```python
from build123d import *

# Parameters (mm, degrees)
SKETCH1_W            = 48
SKETCH1_H            = 53
BOSS_EXTRUDE1_DEPTH  = 10
SKETCH2_W            = 48
SKETCH2_H            = 5.616325
BOSS_EXTRUDE2_DEPTH  = 33.1917878
SKETCH4_W            = 4
SKETCH4_H            = 10
BOSS_EXTRUDE4_DEPTH  = 40
SKETCH5_W            = 48
SKETCH5_H            = 10.8609375
BOSS_EXTRUDE5_DEPTH  = 23.1917878
SKETCH6_W            = 48
SKETCH6_H            = 5
BOSS_EXTRUDE6_DEPTH  = 42.3
SKETCH7_W            = 12.8082122
SKETCH7_H            = 16.4772625
BOSS_EXTRUDE7_DEPTH  = 48
CUT_EXTRUDE1_REACH   = 84.426
SKETCH8_R            = 11.5
SKETCH8_R_2          = 1.5
FILLET1_R            = 10
FILLET2_R            = 4
SKETCH9_W            = 5
SKETCH9_H            = 16.4772625
BOSS_EXTRUDE9_DEPTH  = 48
CUT_EXTRUDE2_DEPTH   = 6
SKETCH11_R           = 1.9304
CUT_EXTRUDE3_DEPTH   = 6
BOSS_EXTRUDE11_DEPTH = 3
SKETCH14_W           = 45
SKETCH14_H           = 17
CUT_EXTRUDE4_DEPTH   = 4
CUT_EXTRUDE5_REACH   = 88.925


with BuildPart() as part:
    # Sketch1 → Boss-Extrude1 (new body)
    with BuildSketch(Plane.XY):
        with Locations((24, 26.5)):
            Rectangle(SKETCH1_W, SKETCH1_H)
    extrude(amount=BOSS_EXTRUDE1_DEPTH)

    # Sketch2 → Boss-Extrude2 (add)
    with BuildSketch(Plane(origin=(0, 0, 0), x_dir=(-1, 0, 0), z_dir=(0, 0, -1))):
        with Locations((-24, -2.8081625)):
            Rectangle(SKETCH2_W, SKETCH2_H)
    extrude(amount=-BOSS_EXTRUDE2_DEPTH)

    # Sketch4 → Boss-Extrude4 (add)
    with BuildSketch(Plane.XY.offset(10)):
        with Locations((2, 48)):
            Rectangle(SKETCH4_W, SKETCH4_H)
        with Locations((46, 48)):
            Rectangle(SKETCH4_W, SKETCH4_H)
    extrude(amount=BOSS_EXTRUDE4_DEPTH)

    # Sketch5 → Boss-Extrude5 (add)
    with BuildSketch(Plane.XY.offset(10)):
        with Locations((24, 5.43046875)):
            Rectangle(SKETCH5_W, SKETCH5_H)
    extrude(amount=BOSS_EXTRUDE5_DEPTH)

    # Sketch6 → Boss-Extrude6 (add)
    with BuildSketch(Plane.XZ.offset(5.616325)):
        with Locations((24, 30.6917878)):
            Rectangle(SKETCH6_W, SKETCH6_H)
    extrude(amount=BOSS_EXTRUDE6_DEPTH)

    # Sketch7 → Boss-Extrude7 (add)
    with BuildSketch(Plane.ZY):
        with Locations((-6.4041061, 2.62230625)):
            Rectangle(SKETCH7_W, SKETCH7_H)
    extrude(amount=-BOSS_EXTRUDE7_DEPTH)

    # Sketch8 → Cut-Extrude1 (cut, up to next)
    with BuildSketch(Plane(origin=(0, 0, 28.1917878), x_dir=(-1, 0, 0), z_dir=(0, 0, -1)), mode=Mode.PRIVATE) as cut_extrude1_sk1:
        with Locations((-24, -26.616325)):
            Circle(SKETCH8_R)
    cut_extrude1_tool1 = extrude(cut_extrude1_sk1.sketch, amount=-CUT_EXTRUDE1_REACH, mode=Mode.PRIVATE) & part.part
    # Sketch8 → Cut-Extrude1 (cut, up to next)
    with BuildSketch(Plane(origin=(0, 0, 28.1917878), x_dir=(-1, 0, 0), z_dir=(0, 0, -1)), mode=Mode.PRIVATE) as cut_extrude1_sk2:
        with Locations((-39.5, -11.116325)):
            Circle(SKETCH8_R_2)
    cut_extrude1_tool2 = extrude(cut_extrude1_sk2.sketch, amount=-CUT_EXTRUDE1_REACH, mode=Mode.PRIVATE) & part.part
    # Sketch8 → Cut-Extrude1 (cut, up to next)
    with BuildSketch(Plane(origin=(0, 0, 28.1917878), x_dir=(-1, 0, 0), z_dir=(0, 0, -1)), mode=Mode.PRIVATE) as cut_extrude1_sk3:
        with Locations((-39.5, -42.116325)):
            Circle(SKETCH8_R_2)
    cut_extrude1_tool3 = extrude(cut_extrude1_sk3.sketch, amount=-CUT_EXTRUDE1_REACH, mode=Mode.PRIVATE) & part.part
    # Sketch8 → Cut-Extrude1 (cut, up to next)
    with BuildSketch(Plane(origin=(0, 0, 28.1917878), x_dir=(-1, 0, 0), z_dir=(0, 0, -1)), mode=Mode.PRIVATE) as cut_extrude1_sk4:
        with Locations((-8.5, -11.116325)):
            Circle(SKETCH8_R_2)
    cut_extrude1_tool4 = extrude(cut_extrude1_sk4.sketch, amount=-CUT_EXTRUDE1_REACH, mode=Mode.PRIVATE) & part.part
    # Sketch8 → Cut-Extrude1 (cut, up to next)
    with BuildSketch(Plane(origin=(0, 0, 28.1917878), x_dir=(-1, 0, 0), z_dir=(0, 0, -1)), mode=Mode.PRIVATE) as cut_extrude1_sk5:
        with Locations((-8.5, -42.116325)):
            Circle(SKETCH8_R_2)
    cut_extrude1_tool5 = extrude(cut_extrude1_sk5.sketch, amount=-CUT_EXTRUDE1_REACH, mode=Mode.PRIVATE) & part.part
    add(cut_extrude1_tool1.solids().sort_by_distance((24, -26.616325, 28.191788))[0], mode=Mode.SUBTRACT)
    add(cut_extrude1_tool2.solids().sort_by_distance((39.5, -11.116325, 28.191788))[0], mode=Mode.SUBTRACT)
    add(cut_extrude1_tool3.solids().sort_by_distance((39.5, -42.116325, 28.191788))[0], mode=Mode.SUBTRACT)
    add(cut_extrude1_tool4.solids().sort_by_distance((8.5, -11.116325, 28.191788))[0], mode=Mode.SUBTRACT)
    add(cut_extrude1_tool5.solids().sort_by_distance((8.5, -42.116325, 28.191788))[0], mode=Mode.SUBTRACT)

    # Fillet1
    fillet1_edges = [part.edges().sort_by_distance(p)[0] for p in [
        (24, 10.8609375, 0),
    ]]
    fillet(fillet1_edges, radius=FILLET1_R)

    # Fillet2
    fillet2_edges = [part.edges().sort_by_distance(p)[0] for p in [
        (2, 43, 10),
        (46, 43, 10),
    ]]
    fillet(fillet2_edges, radius=FILLET2_R)

    # Sketch9 → Boss-Extrude9 (add)
    with BuildSketch(Plane(origin=(48, 0, 0), x_dir=(0, 0, -1), z_dir=(1, 0, 0))):
        with Locations((15.3082122, 2.62230625)):
            Rectangle(SKETCH9_W, SKETCH9_H)
    extrude(amount=-BOSS_EXTRUDE9_DEPTH)

    # Sketch10 → Cut-Extrude2 (cut)
    with BuildSketch(Plane.XY.offset(10)):
        Polygon((7.020265927, 38.429), (5.040531854, 35), (7.020265927, 31.571), (10.979734073, 31.571), (12.959468146, 35), (10.979734073, 38.429), align=None)
        Polygon((37.020265927, 31.571), (40.979734073, 31.571), (42.959468146, 35), (40.979734073, 38.429), (37.020265927, 38.429), (35.040531854, 35), align=None)
    extrude(amount=-CUT_EXTRUDE2_DEPTH, mode=Mode.SUBTRACT)

    # Sketch11 → Cut-Extrude3 (cut)
    with BuildSketch(Plane.XY.offset(4)):
        with Locations((9, 35)):
            Circle(SKETCH11_R)
        with Locations((39, 35)):
            Circle(SKETCH11_R)
    extrude(amount=-CUT_EXTRUDE3_DEPTH, mode=Mode.SUBTRACT)

    # Sketch12 → Boss-Extrude11 (add)
    with BuildSketch(Plane(origin=(0, 53, 0), x_dir=(1, 0, 0), z_dir=(0, 1, 0))):
        Polygon((0, 0), (0, -50), (4, -50), (4, -10), (44, -10), (44, -50), (48, -50), (48, 0), align=None)
    extrude(amount=BOSS_EXTRUDE11_DEPTH)

    # Sketch14 → Cut-Extrude4 (cut)
    with BuildSketch(Plane.ZY):
        with Locations((27.5, 47.5)):
            Rectangle(SKETCH14_W, SKETCH14_H)
    extrude(amount=-CUT_EXTRUDE4_DEPTH, mode=Mode.SUBTRACT)

    # Sketch15 → Cut-Extrude5 (cut, up to next)
    with BuildSketch(Plane(origin=(0, 0, 28.1917878), x_dir=(-1, 0, 0), z_dir=(0, 0, -1)), mode=Mode.PRIVATE) as cut_extrude5_sk1:
        with BuildLine():
            Line((-10.43028611, -26.616325), (-13.577258578, -21.756647928))
            ThreePointArc((-13.577258578, -21.756647928), (-12.772544225, -24.127502624), (-12.5, -26.616325))
            ThreePointArc((-12.5, -26.616325), (-12.772544225, -29.105147376), (-13.577258578, -31.476002072))
            Line((-13.577258578, -31.476002072), (-10.43028611, -26.616325))
        make_face()
    cut_extrude5_tool1 = extrude(cut_extrude5_sk1.sketch, amount=-CUT_EXTRUDE5_REACH, mode=Mode.PRIVATE) & part.part
    # Sketch15 → Cut-Extrude5 (cut, up to next)
    with BuildSketch(Plane(origin=(0, 0, 28.1917878), x_dir=(-1, 0, 0), z_dir=(0, 0, -1)), mode=Mode.PRIVATE) as cut_extrude5_sk2:
        with BuildLine():
            Line((-6.602022713, -11.116325), (-7.2091403, -10.352334664))
            ThreePointArc((-7.2091403, -10.352334664), (-7.053229536, -10.720275477), (-7, -11.116325))
            ThreePointArc((-7, -11.116325), (-7.053229536, -11.512374523), (-7.2091403, -11.880315336))
            Line((-7.2091403, -11.880315336), (-6.602022713, -11.116325))
        make_face()
    cut_extrude5_tool2 = extrude(cut_extrude5_sk2.sketch, amount=-CUT_EXTRUDE5_REACH, mode=Mode.PRIVATE) & part.part
    # Sketch15 → Cut-Extrude5 (cut, up to next)
    with BuildSketch(Plane(origin=(0, 0, 28.1917878), x_dir=(-1, 0, 0), z_dir=(0, 0, -1)), mode=Mode.PRIVATE) as cut_extrude5_sk3:
        with BuildLine():
            Line((-37.602022713, -11.116325), (-38.2091403, -10.352334664))
            ThreePointArc((-38.2091403, -10.352334664), (-38.053229536, -10.720275477), (-38, -11.116325))
            ThreePointArc((-38, -11.116325), (-38.053229536, -11.512374523), (-38.2091403, -11.880315336))
            Line((-38.2091403, -11.880315336), (-37.602022713, -11.116325))
        make_face()
    cut_extrude5_tool3 = extrude(cut_extrude5_sk3.sketch, amount=-CUT_EXTRUDE5_REACH, mode=Mode.PRIVATE) & part.part
    # Sketch15 → Cut-Extrude5 (cut, up to next)
    with BuildSketch(Plane(origin=(0, 0, 28.1917878), x_dir=(-1, 0, 0), z_dir=(0, 0, -1)), mode=Mode.PRIVATE) as cut_extrude5_sk4:
        with BuildLine():
            Line((-37.602022713, -42.116325), (-38.2091403, -41.352334664))
            ThreePointArc((-38.2091403, -41.352334664), (-38.053229536, -41.720275477), (-38, -42.116325))
            ThreePointArc((-38, -42.116325), (-38.053229536, -42.512374523), (-38.2091403, -42.880315336))
            Line((-38.2091403, -42.880315336), (-37.602022713, -42.116325))
        make_face()
    cut_extrude5_tool4 = extrude(cut_extrude5_sk4.sketch, amount=-CUT_EXTRUDE5_REACH, mode=Mode.PRIVATE) & part.part
    # Sketch15 → Cut-Extrude5 (cut, up to next)
    with BuildSketch(Plane(origin=(0, 0, 28.1917878), x_dir=(-1, 0, 0), z_dir=(0, 0, -1)), mode=Mode.PRIVATE) as cut_extrude5_sk5:
        with BuildLine():
            Line((-6.602022713, -42.116325), (-7.2091403, -41.352334664))
            ThreePointArc((-7.2091403, -41.352334664), (-7.053229536, -41.720275477), (-7, -42.116325))
            ThreePointArc((-7, -42.116325), (-7.053229536, -42.512374523), (-7.2091403, -42.880315336))
            Line((-7.2091403, -42.880315336), (-6.602022713, -42.116325))
        make_face()
    cut_extrude5_tool5 = extrude(cut_extrude5_sk5.sketch, amount=-CUT_EXTRUDE5_REACH, mode=Mode.PRIVATE) & part.part
    add(cut_extrude5_tool1.solids().sort_by_distance((12.00141, -26.616325, 28.191788))[0], mode=Mode.SUBTRACT)
    add(cut_extrude5_tool2.solids().sort_by_distance((6.903574, -11.116325, 28.191788))[0], mode=Mode.SUBTRACT)
    add(cut_extrude5_tool3.solids().sort_by_distance((37.903574, -11.116325, 28.191788))[0], mode=Mode.SUBTRACT)
    add(cut_extrude5_tool4.solids().sort_by_distance((37.903574, -42.116325, 28.191788))[0], mode=Mode.SUBTRACT)
    add(cut_extrude5_tool5.solids().sort_by_distance((6.903574, -42.116325, 28.191788))[0], mode=Mode.SUBTRACT)


solid = part.part
```
The model under review builds one solid part; all positions refer to its coordinate system, in mm. A direction names the side the tool comes from. Round coordinates to 2 decimals unless told otherwise and drop trailing zeros. Loops run counter-clockwise (first coordinate to the right, second up) from the corner with the lowest first, then second, coordinate; pieces in that order, holes last. Notation, with made-up numbers: (-24, -36) - (28, -36) arc R23 cw to (28, -17) - close; hole circle Ø1 at (15, 39). An arc over 180 degrees is marked (long way). Use a Markdown table: item, result. Add a question column.
Q1. The part is to be moulded in two halves that separate along Y. For faces 1 (the face through (41, -11.1, 30.7)), 2 (the face through (24.34, 13.71, -3.01)), 3 (the face through (44, 49, 30)), say which applies: pulls with the +Y half, pulls with the -Y half, needs draft (parallel to the pull), parting line crosses it, or undercut.
Q2. Add section A-A (z = 22). State the section outline as (x, y) points.
Q3. Add section C-C (y = 48). State the section outline as (x, z) points.
Q4. Insertion check: pin 1 Ø7 at (x, z) = (21, 24.5) entering from +Y; pin 2 Ø5.5 at (x, y) = (40, 35.5) entering from +Z; pin 3 Ø3.5 at (x, y) = (10, 36.5) entering from +Z. Each pin has a flat end and moves straight along its axis. Give the tip position at first contact, or say it passes through.
Q5. Add section B-B (x = 28). State the section outline as (y, z) points, plus the area to 3 significant figures.
Q6. Add section D-D (x = 39.5). State the section outline as (y, z) points, plus the area to 3 significant figures.
Q7. Machinability: for faces 4 (the face through (46.028, 41.797, 11.141)), 5 (the face through (11.98, -24.22, 30.66)), 6 (the face through (2, 47, 5)), 7 (the face through (6.044, 36.739, 7.042)), which of the approach directions +Z, -Z, +X, -X, +Y, -Y give a long, thin tool a straight path to every point of the face, cutting with its end or side? Answer none if there is none.
Q8. For probe 1 along Y at (x, z) = (24, 31); probe 2 along Y at (x, z) = (9, 1.15); probe 3 along Z at (x, y) = (21, 2), list the stretches that pass through material, from the lowest coordinate up.
Worked answers:
| question | item | result |
|---|---|---|
| 1 | face 1 | undercut |
| 1 | face 2 | pulls with the +Y half |
| 1 | face 3 | needs draft |
| 2 | outline | (0, -5.62) - (48, -5.62) - (48, 10.86) - (0, 10.86) - close; (44, 43) - (48, 43) - (48, 56) - (44, 56) - close |
| 3 | outline | (0, 0) - (48, 0) - (48, 50) - (44, 50) - (44, 10) - (4, 10) - (4, 5) - (0, 5) - close |
| 4 | pin 1 | y = 10.86 |
| 4 | pin 2 | z = 10 |
| 4 | pin 3 | z = 4 |
| 5 | outline | (-47.92, 28.19) - (-37.4, 28.19) - (-37.4, 33.19) - (-47.92, 33.19) - close; (-15.83, 28.19) - (-5.62, 28.19) - (-5.62, -17.81) - (10.86, -17.81) - (10.86, -10) arc R10 cw to (20.86, 0) - (56, 0) - (56, 10) - (10.86, 10) - (10.86, 33.19) - (-15.83, 33.19) - close |
| 5 | area | 1,420 mm² |
| 6 | outline | (-47.92, 28.19) - (-43.62, 28.19) - (-43.62, 33.19) - (-47.92, 33.19) - close; (-40.62, 28.19) - (-12.62, 28.19) - (-12.62, 33.19) - (-40.62, 33.19) - close; (-9.62, 28.19) - (-5.62, 28.19) - (-5.62, -17.81) - (10.86, -17.81) - (10.86, -10) arc R10 cw to (20.86, 0) - (33.14, 0) - (33.14, 4) - (31.57, 4) - (31.57, 10) - (10.86, 10) - (10.86, 33.19) - (-9.62, 33.19) - close; (36.86, 0) - (56, 0) - (56, 10) - (38.43, 10) - (38.43, 4) - (36.86, 4) - close |
| 6 | area | 1,440 mm² |
| 7 | face 4 | +Z, +X, -X |
| 7 | face 5 | +Z, -Z |
| 7 | face 6 | +Z, -X, +Y |
| 7 | face 7 | +Z |
| 8 | probe 1 | -47.92 to -38.12, -15.12 to 10.86 |
| 8 | probe 2 | -5.62 to 33.07, 36.93 to 56 |
| 8 | probe 3 | -17.81 to 33.19 |
